Model file for the job. Use its own axes, mm. Face numbers are marked on the shaded views. A direction names the side the tool comes from. Round coordinates to 2 decimals unless told otherwise and drop trailing zeros. Loops run counter-clockwise (first coordinate to the right, second up) from the corner with the lowest first, then second, coordinate; pieces in that order, holes last. Notation, with made-up numbers: M 62,-3.5 L 114,-3.5 A24 ccw 114,28.5 Z; hole C 38,-30.5 d3. An arc over 180 degrees is marked long. Use a Markdown table: item, result. Add a question column.
Q1. Cut at C-C (x = 195.5). Give the cut face in (y, z), plus the area to 3 significant figures.
Q2. Cut at A-A (z = 0). Give the cut face in (x, y), plus the area to 3 significant figures.
Q3. Pin check, flat tips, straight feed: pin 1 (1.2 mm diameter, centred on y = -0.5, z = -28.5, fed in from +X); pin 2 (12 mm diameter, centred on y = 8, z = 6, fed in from +X); pin 3 (8 mm diameter, centred on x = 245.7, y = 0, fed in from +Z). Stop position of each tip, or through.
Q4. Tool access for the marked faces 1, 2 and 3: list every direction of +Z, -Z, +X, -X, +Y, -Y with a clear straight run to the whole face (end or side of a thin tool).
Q5. Probe line 1 (X direction, y = 0, z = 31); line 2 (X direction, y = 0, z = 28); line 3 (Z direction, x = 94, y = 0). List the from-to ranges inside material, lowest first. Write a range as from..to.
Q6. Mould opens along Z. For the marked faces 4, 5 and 6 say: +Z half, -Z half, draft (parallel to the pull), parting line (faces both ways), or undercut.
Q7. Cut at B-B (y = 0). State how many separate pieces and enclosed holes the cut face has, plus the area to 3 significant figures.
from build123d import *

# Parameters (mm, degrees)
F4_DEPTH    = 15
F5_T1_DEPTH = 27.5
F5_T4_ANGLE = 180
F5_T6_ANGLE = 180
F7_R        = 8
F7_R_2      = 5
F9_D        = 6
F9_DEPTH    = 20
F9_START    = 6.1555899
F9_TIP      = 1.8025818571
F10_D       = 6
F10_DEPTH   = 20
F10_START   = 6.1555899
F10_TIP     = 1.8025818571


# Not quite as in the source:
# - a fillet or chamfer that OpenCascade refuses, or shapes differently, is made with other operations: its cross-section is extruded or revolved along the edge and cut away or added


with BuildPart() as f3:
    # F2 (on Front) → F3 (revolve)
    with BuildSketch(Plane.XZ):
        Polygon((105.0486442498, 29), (98.7043133404, 29), (98.7043133404, 25.5), (105.7043133404, 25.5), (107.0780520501, 25), (250.7043133404, 25), (250.7043133404, 0), (260.7043133404, 0), (260.7043133404, 27.5), (260.7043133404, 29), align=None)
        Polygon((92.3599824309, 29), (60.7043133404, 29), (60.7043133404, 26.6542383736), (79.2043133404, 26.6542383736), (81.2035128474, 25.5), (98.7043133404, 25.5), (98.7043133404, 29), align=None)
    revolve(axis=Axis((125.4885941744, 0, 0), (1, 0, 0)))

    # F2 (on Front) → F4 (join, symmetric)
    with BuildSketch(Plane.XZ):
        with BuildLine():
            Line((288.2043133404, 27.5), (260.7043133404, 27.5))
            Line((260.7043133404, 27.5), (260.7043133404, 0))
            Line((260.7043133404, 0), (260.7043133404, -27.5))
            Line((260.7043133404, -27.5), (288.2043133404, -27.5))
            ThreePointArc((288.2043133404, -27.5), (315.7043133404, 0), (288.2043133404, 27.5))
        make_face()
        with BuildLine():
            ThreePointArc((303.2043133404, 0), (288.2043133404, -15), (273.2043133404, 0))
            ThreePointArc((273.2043133404, 0), (288.2043133404, 15), (303.2043133404, 0))
        make_face(mode=Mode.SUBTRACT)
    extrude(amount=F4_DEPTH, both=True)

    # F5: chamfer of 5 on 6 edges, made by hand

    # F5_s2 → F5_t1 (cut)
    with BuildSketch(Plane.YZ.offset(260.7043133404)):
        Polygon((-10, 27.5), (-15, 22.5), (-15, 27.5), align=None)
        Polygon((10, 27.5), (15, 22.5), (15, 27.5), align=None)
        Polygon((15, -22.5), (10, -27.5), (15, -27.5), align=None)
        Polygon((-10, -27.5), (-15, -22.5), (-15, -27.5), align=None)
    extrude(amount=F5_T1_DEPTH, mode=Mode.SUBTRACT)

    # F5_s3 → F5_t4 (revolve, cut)
    with BuildSketch(Plane.YZ.offset(288.2043133404)):
        Polygon((15, -22.5), (10, -27.5), (15, -27.5), align=None)
    revolve(axis=Axis((288.2043133404, 15, 0), (0, -1, 0)), revolution_arc=F5_T4_ANGLE, mode=Mode.SUBTRACT)

    # F5_s5 → F5_t6 (revolve, cut)
    with BuildSketch(Plane.YZ.offset(288.2043133404)):
        Polygon((-15, -22.5), (-10, -27.5), (-15, -27.5), align=None)
    revolve(axis=Axis((288.2043133404, -15, 0), (0, -1, 0)), revolution_arc=F5_T6_ANGLE, mode=Mode.SUBTRACT)

    # F7 (on offset) → F8 (join, up to the next surface of F3)
    with BuildSketch(Plane.XY.offset(35)):
        with Locations((98.7043133404, 0)):
            Circle(F7_R)
        with Locations((98.7043133404, 0)):
            Circle(F7_R_2, mode=Mode.SUBTRACT)
        with Locations((245.7043133404, 0)):
            Circle(F7_R)
        with Locations((245.7043133404, 0)):
            Circle(F7_R_2, mode=Mode.SUBTRACT)
    extrude(until=Until.NEXT, dir=(0, 0, -1))

    # F9
    # its depths count from where the whole tool has entered the part; down to there all is cleared
    with Locations(Plane.XY.offset(35).offset(-F9_START)):
        with Locations((98.7043133404, 0)):
            Hole(F9_D / 2, depth=F9_DEPTH)
            with Locations((0, 0, -(F9_DEPTH + F9_TIP / 2))):  # 118° drill point
                Cone(0, F9_D / 2, F9_TIP, mode=Mode.SUBTRACT)

    # F10
    # its depths count from where the whole tool has entered the part; down to there all is cleared
    with Locations(Plane.XY.offset(35).offset(-F10_START)):
        with Locations((245.7043133404, 0)):
            Hole(F10_D / 2, depth=F10_DEPTH)
            with Locations((0, 0, -(F10_DEPTH + F10_TIP / 2))):  # 118° drill point
                Cone(0, F10_D / 2, F10_TIP, mode=Mode.SUBTRACT)


solid = f3.part
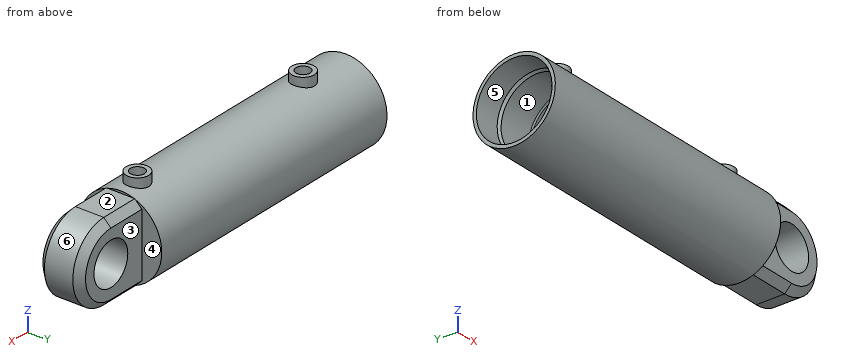
Checked values:
| question | item | result |
|---|---|---|
| 1 | outline | C 0,0 d58; hole C 0,0 d50 |
| 1 | area | 679 mm^2 |
| 2 | outline | M 60.7,-29 L 260.7,-29 L 260.7,-15 L 273.2,-15 L 273.2,15 L 260.7,15 L 260.7,29 L 60.7,29 L 60.7,26.65 L 79.2,26.65 L 81.2,25.5 L 105.7,25.5 L 107.08,25 L 250.7,25 L 250.7,-25 L 107.08,-25 L 105.7,-25.5 L 81.2,-25.5 L 79.2,-26.65 L 60.7,-26.65 Z; M 303.2,-15 L 310.7,-15 L 315.7,-10 L 315.7,10 L 310.7,15 L 303.2,15 Z |
| 2 | area | 2,730 mm^2 |
| 3 | pin 1 | stops at x = 260.7 |
| 3 | pin 2 | stops at x = 315.7 |
| 3 | pin 3 | stops at z = 29 |
| 4 | face 1 | -X |
| 4 | face 2 | +Z, +X, +Y, -Y |
| 4 | face 3 | +Z, -Z, +X, +Y |
| 5 | line 1 | x = 90.7..93.7, 103.7..106.7, 237.7..240.7, 250.7..253.7 |
| 5 | line 2 | x = 60.7..95.7, 101.7..242.7, 248.7..260.7 |
| 5 | line 3 | z = -29..-25.5, 25.5..29 |
| 6 | face 4 | draft |
| 6 | face 5 | undercut |
| 6 | face 6 | parting line |
| 7 | separate pieces | 3 |
| 7 | enclosed holes | 1 |
| 7 | area | 4,030 mm^2 |
